For this review, take the finished solid that the model builds, in its own axes (mm). A direction names the side the tool comes from. Coordinates: 2 decimals unless noted, no trailing zeros. Order: outer loops, then holes, each group sorted by start corner. A loop starts at its lowest first (then second) coordinate and runs counter-clockwise, first axis right, second up.
from build123d import *

# Parameters (mm, degrees)
SKETCH1_W                   = 82.55
SKETCH1_H                   = 101.6
BOSS_EXTRUDE1_DEPTH         = 1.5875
SKETCH2_W                   = 49.2125
SKETCH2_H                   = 69.85
BOSS_EXTRUDE2_DEPTH         = 28.575
SKETCH3_R                   = 3.175
BOSS_EXTRUDE3_DEPTH         = 34.925
F_1_4_0_25_DIAMETER_HOLE1_D = 6.35
SKETCH6_W                   = 38.1
SKETCH6_H                   = 63.5
CUT_EXTRUDE1_DEPTH          = 31.1625


with BuildPart() as part:
    # Sketch1 → Boss-Extrude1 (new body)
    with BuildSketch(Plane.XY):
        Rectangle(SKETCH1_W, SKETCH1_H)
    extrude(amount=BOSS_EXTRUDE1_DEPTH)

    # Sketch2 → Boss-Extrude2 (add)
    with BuildSketch(Plane.XY.offset(1.5875)):
        Rectangle(SKETCH2_W, SKETCH2_H)
    extrude(amount=BOSS_EXTRUDE2_DEPTH)

    # Sketch3 → Boss-Extrude3 (add)
    with BuildSketch(Plane.XY.offset(1.5875)):
        with Locations((-24.60625, 25.4)):
            Circle(SKETCH3_R)
        with Locations((24.60625, 25.4)):
            Circle(SKETCH3_R)
        with Locations((-24.60625, -25.4)):
            Circle(SKETCH3_R)
        with Locations((24.60625, -25.4)):
            Circle(SKETCH3_R)
    extrude(amount=BOSS_EXTRUDE3_DEPTH)

    # 1/4 (0.25) Diameter Hole1 (through all)
    with Locations(Plane.XY.offset(1.5875)):
        with Locations((-27.78125, 42.8625), (27.78125, 42.8625), (-27.78125, -42.8625), (27.78125, -42.8625)):
            Hole(F_1_4_0_25_DIAMETER_HOLE1_D / 2)

    # Sketch6 → Cut-Extrude1 (cut, through all)
    with BuildSketch(Plane.XY.offset(30.1625)):
        Rectangle(SKETCH6_W, SKETCH6_H)
    extrude(amount=-CUT_EXTRUDE1_DEPTH, mode=Mode.SUBTRACT)


solid = part.part
1. Machinability: for faces 4 (the face through (-24.606, -32, 16)), 5 (the face through (19.05, 0, 15)), 6 (the face through (-24.606, 32, 16)), 7 (the face through (24.606, 32, 16)), 8 (the face through (-24.606, 0, 16)), which of the approach directions +Z, -Z, +X, -X, +Y, -Y give a long, thin tool a straight path to every point of the face, cutting with its end or side? Answer none if there is none.
Answer below:
face 4: +Z, -X, -Y
face 5: +Z, -Z
face 6: +Z, -X, +Y
face 7: +Z, +X, +Y
face 8: +Z, -X
2. To check wall thickness, follow L1, parallel to X at y = -25, z = 29; L2, parallel to X at y = -19.5, z = 28; L3, parallel to Y at x = 18.5, z = 12 (3 decimals). State the ranges of each line that lie inside material, in increasing order.
Answer below:
L1: x = -27.76 to -19.05, 19.05 to 27.76
L2: x = -24.61 to -19.05, 19.05 to 24.61
L3: y = -34.925 to -31.75, 31.75 to 34.925
3. Take a section at B-B, the plane z = 10.5. Give the boundary of the cut face in (x, y) (3 decimals).
Answer below:
outline: (-24.606, -34.925) - (24.606, -34.925) - (24.606, -28.575) arc R3.175 ccw to (24.606, -22.225) - (24.606, 22.225) arc R3.175 ccw to (24.606, 28.575) - (24.606, 34.925) - (-24.606, 34.925) - (-24.606, 28.575) arc R3.175 ccw to (-24.606, 22.225) - (-24.606, -22.225) arc R3.175 ccw to (-24.606, -28.575) - close; hole (-19.05, -31.75) - (19.05, -31.75) - (19.05, 31.75) - (-19.05, 31.75) - close
4. The part is to be moulded in two halves that separate along Y. For faces 1 (the face through (24.606, 0, 16)), 2 (the face through (25, 25, 36.512)), 3 (the face through (0, 34.925, 16)), say which applies: +Y half, -Y half, draft (parallel to the pull), parting line (faces both ways), or undercut.
Answer below:
face 1: undercut
face 2: draft
face 3: +Y half
5. Clearance check with flat-ended pins moving along their axes: pin 1 Ø4 at (x, y) = (-27.78, 42.86) entering from -Z; pin 2 Ø8 at (x, z) = (11.5, 11) entering from -Y (3 decimals); pin 3 Ø7.5 at (x, y) = (-27.78, -42.86) entering from +Z; pin 4 Ø6 at (y, z) = (33, 30.5) entering from +X. State where each tip first meets the part, or that it passes through.
Answer below:
pin 1: passes through
pin 2: stops at y = -34.925
pin 3: stops at z = 1.59
pin 4: stops at x = 24.61
